```python
from build123d import *

# Parameters (mm, degrees)
BASE_FLANGE1_DEPTH    = 1
EDGE_FLANGE2_DEPTH    = 85
EDGE_FLANGE3_DEPTH    = 192.5
EDGE_FLANGE1_DEPTH    = 65
EDGE_FLANGE4_DEPTH    = 77.781745931
EDGE_FLANGE5_DEPTH    = 30
BREAK_CORNER1_START   = 128
BREAK_CORNER1_DEPTH   = 69
BREAK_CORNER1_START_2 = 196
BREAK_CORNER1_2_DEPTH = 1
BREAK_CORNER1_START_3 = -150.492424049
BREAK_CORNER1_3_DEPTH = 1
BREAK_CORNER1_START_4 = -2
BREAK_CORNER1_4_DEPTH = 19
BREAK_CORNER1_START_5 = 16
BREAK_CORNER1_5_DEPTH = 1
BREAK_CORNER1_6_DEPTH = 1
BREAK_CORNER1_START_6 = -1
BREAK_CORNER1_7_DEPTH = 1
CUT_EXTRUDE1_REACH    = 150.327


# Read off the part's stored shape, not the designer's step: Break-Corner1
# Sheet-metal steps are written as plain solids
with BuildPart() as part:
    # Sketch1 → Base-Flange1 (new body)
    with BuildSketch(Plane.XY):
        Polygon((0, 130), (-70, 130), (-70, 140), (-15, 195), (15, 195), (15, 130), (15, 0), (0, 0), align=None)
    extrude(amount=-BASE_FLANGE1_DEPTH)

    # Edge-Flange2 section (across the edge) → Edge-Flange2 (add)
    with BuildSketch(Plane(origin=(-1, 2.5, -1), x_dir=(1, 0, 0), z_dir=(0, 1, 0))):
        with BuildLine():
            Line((-1, 1), (-1, 12))
            Line((-1, 12), (0, 12))
            Line((0, 12), (0, 1))
            ThreePointArc((0, 1), (0.292893219, 0.292893219), (1, 0))
            Line((1, 0), (1, -1))
            ThreePointArc((1, -1), (-0.414213562, -0.414213562), (-1, 1))
        make_face()
    extrude(amount=EDGE_FLANGE2_DEPTH)

    # Edge-Flange3 section (across the edge) → Edge-Flange3 (add)
    with BuildSketch(Plane(origin=(16, 195, -1), x_dir=(-1, 0, 0), z_dir=(0, -1, 0))):
        with BuildLine():
            Line((-1, 1), (-1, 10))
            Line((-1, 10), (0, 10))
            Line((0, 10), (0, 1))
            ThreePointArc((0, 1), (0.292893219, 0.292893219), (1, 0))
            Line((1, 0), (1, -1))
            ThreePointArc((1, -1), (-0.414213562, -0.414213562), (-1, 1))
        make_face()
    extrude(amount=EDGE_FLANGE3_DEPTH)

    # Edge-Flange1 section (across the edge) → Edge-Flange1 (add)
    with BuildSketch(Plane(origin=(-2.5, 129, -1), x_dir=(0, 1, 0), z_dir=(-1, 0, 0))):
        with BuildLine():
            Line((-1, 1), (-1, 15.122069622))
            Line((-1, 15.122069622), (0, 15.122069622))
            Line((0, 15.122069622), (0, 1))
            ThreePointArc((0, 1), (0.292893219, 0.292893219), (1, 0))
            Line((1, 0), (1, -1))
            ThreePointArc((1, -1), (-0.414213562, -0.414213562), (-1, 1))
        make_face()
    extrude(amount=EDGE_FLANGE1_DEPTH)

    # Edge-Flange4 section (across the edge) → Edge-Flange4 (add)
    with BuildSketch(Plane(origin=(-70.707106781, 140.707106781, -1), x_dir=(0.7071067811865439, -0.7071067811865512, -3.4914813388431337e-15), z_dir=(0.7071067811865512, 0.7071067811865439, 0))):
        with BuildLine():
            Line((-1, 1), (-1, 10))
            Line((-1, 10), (0, 10))
            Line((0, 10), (0, 1))
            ThreePointArc((0, 1), (0.292893219, 0.292893219), (1, 0))
            Line((1, 0), (1, -1))
            ThreePointArc((1, -1), (-0.414213562, -0.414213562), (-1, 1))
        make_face()
    extrude(amount=EDGE_FLANGE4_DEPTH)

    # Edge-Flange5 section (across the edge) → Edge-Flange5 (add)
    with BuildSketch(Plane(origin=(-15, 196, -1), x_dir=(0, -1, 0), z_dir=(1, 0, 0))):
        with BuildLine():
            Line((-1, 1), (-1, 10))
            Line((-1, 10), (0, 10))
            Line((0, 10), (0, 1))
            ThreePointArc((0, 1), (0.292893219, 0.292893219), (1, 0))
            Line((1, 0), (1, -1))
            ThreePointArc((1, -1), (-0.414213562, -0.414213562), (-1, 1))
        make_face()
    extrude(amount=EDGE_FLANGE5_DEPTH)

    # Break-Corner1 outline → Break-Corner1 (cut)
    with BuildSketch(Plane(origin=(0, 0, 0), x_dir=(1, 0, 0), z_dir=(0, 1, 0)).offset(BREAK_CORNER1_START)):
        with BuildLine():
            ThreePointArc((-67.5, 13.622069622), (-66.767766953, 15.389836575), (-65, 16.122069622))
            Line((-65, 16.122069622), (-67.5, 16.122069622))
            Line((-67.5, 16.122069622), (-67.5, 13.622069622))
        make_face()
        with BuildLine():
            ThreePointArc((-5, 16.122069622), (-3.232233047, 15.389836575), (-2.5, 13.622069622))
            Line((-2.5, 13.622069622), (-2.5, 16.122069622))
            Line((-2.5, 16.122069622), (-5, 16.122069622))
        make_face()
        with BuildLine():
            Line((15, 11), (12.5, 11))
            ThreePointArc((12.5, 11), (14.267766953, 10.267766953), (15, 8.5))
            Line((15, 8.5), (15, 11))
        make_face()
    extrude(amount=BREAK_CORNER1_DEPTH, mode=Mode.SUBTRACT)

    # Break-Corner1 2 outline → Break-Corner1 2 (cut)
    with BuildSketch(Plane(origin=(0, 0, 0), x_dir=(1, 0, 0), z_dir=(0, 1, 0)).offset(BREAK_CORNER1_START_2)):
        with BuildLine():
            Line((-15, 11), (-15, 8.5))
            ThreePointArc((-15, 8.5), (-14.267766953, 10.267766953), (-12.5, 11))
            Line((-12.5, 11), (-15, 11))
        make_face()
    extrude(amount=BREAK_CORNER1_2_DEPTH, mode=Mode.SUBTRACT)

    # Break-Corner1 3 outline → Break-Corner1 3 (cut)
    with BuildSketch(Plane(origin=(0, 0, 0), x_dir=(0.7071067811865509, 0.707106781186544, 0), z_dir=(0.707106781186544, -0.707106781186551, 0)).offset(BREAK_CORNER1_START_3)):
        with BuildLine():
            Line((49.497474683, -11), (51.997474683, -11))
            ThreePointArc((51.997474683, -11), (50.22970773, -10.267766953), (49.497474683, -8.5))
            Line((49.497474683, -8.5), (49.497474683, -11))
        make_face()
        with BuildLine():
            ThreePointArc((127.279220614, -8.5), (126.546987567, -10.267766953), (124.779220614, -11))
            Line((124.779220614, -11), (127.279220614, -11))
            Line((127.279220614, -11), (127.279220614, -8.5))
        make_face()
    extrude(amount=BREAK_CORNER1_3_DEPTH, mode=Mode.SUBTRACT)

    # Break-Corner1 4 outline → Break-Corner1 4 (cut)
    with BuildSketch(Plane.YZ.offset(BREAK_CORNER1_START_4)):
        with BuildLine():
            ThreePointArc((195, -8.5), (194.267766953, -10.267766953), (192.5, -11))
            Line((192.5, -11), (195, -11))
            Line((195, -11), (195, -8.5))
        make_face()
        with BuildLine():
            ThreePointArc((87.449489743, -11), (86.58113883, -12.436491673), (85, -13))
            Line((85, -13), (87.5, -13))
            Line((87.5, -13), (87.5, -11))
            Line((87.5, -11), (87.449489743, -11))
        make_face()
        with BuildLine():
            Line((2.5, -13), (5, -13))
            ThreePointArc((5, -13), (3.232233047, -12.267766953), (2.5, -10.5))
            Line((2.5, -10.5), (2.5, -13))
        make_face()
    extrude(amount=BREAK_CORNER1_4_DEPTH, mode=Mode.SUBTRACT)

    # Break-Corner1 5 outline → Break-Corner1 5 (cut)
    with BuildSketch(Plane.YZ.offset(BREAK_CORNER1_START_5)):
        with BuildLine():
            Line((2.550510257, -11), (5, -11))
            ThreePointArc((5, -11), (3.232233047, -10.267766953), (2.5, -8.5))
            Line((2.5, -8.5), (2.5, -10.5))
            ThreePointArc((2.5, -10.5), (2.512659617, -10.751272405), (2.550510257, -11))
        make_face()
    extrude(amount=BREAK_CORNER1_5_DEPTH, mode=Mode.SUBTRACT)

    # Break-Corner1 6 outline → Break-Corner1 6 (cut)
    with BuildSketch(Plane.YZ.offset(BREAK_CORNER1_START_4)):
        with BuildLine():
            ThreePointArc((87.5, -10.5), (87.487340383, -10.751272405), (87.449489743, -11))
            Line((87.449489743, -11), (87.5, -11))
            Line((87.5, -11), (87.5, -10.5))
        make_face()
    extrude(amount=BREAK_CORNER1_6_DEPTH, mode=Mode.SUBTRACT)

    # Break-Corner1 7 outline → Break-Corner1 7 (cut)
    with BuildSketch(Plane.XY.offset(BREAK_CORNER1_START_6)):
        with BuildLine():
            ThreePointArc((-67.5, 130), (-69.267766953, 130.732233047), (-70, 132.5))
            Line((-70, 132.5), (-70, 130))
            Line((-70, 130), (-67.5, 130))
        make_face()
        with BuildLine():
            Line((0, 0), (2.5, 0))
            ThreePointArc((2.5, 0), (0.732233047, 0.732233047), (0, 2.5))
            Line((0, 2.5), (0, 0))
        make_face()
        with BuildLine():
            ThreePointArc((15, 2.5), (14.267766953, 0.732233047), (12.5, 0))
            Line((12.5, 0), (15, 0))
            Line((15, 0), (15, 2.5))
        make_face()
    extrude(amount=BREAK_CORNER1_7_DEPTH, mode=Mode.SUBTRACT)

    # Sketch15 → Cut-Extrude1 (cut, up to next)
    with BuildSketch(Plane(origin=(0, 129, 0), x_dir=(1, 0, 0), z_dir=(0, 1, 0)), mode=Mode.PRIVATE) as cut_extrude1_sk1:
        with BuildLine():
            Line((-60, 10.872069622), (-10, 10.872069622))
            ThreePointArc((-10, 10.872069622), (-8.25, 9.122069622), (-10, 7.372069622))
            Line((-10, 7.372069622), (-60, 7.372069622))
            ThreePointArc((-60, 7.372069622), (-61.75, 9.122069622), (-60, 10.872069622))
        make_face()
    cut_extrude1_tool1 = extrude(cut_extrude1_sk1.sketch, amount=-CUT_EXTRUDE1_REACH, mode=Mode.PRIVATE) & part.part
    add(cut_extrude1_tool1.solids().sort_by_distance((-35, 129, -9.12207))[0], mode=Mode.SUBTRACT)


solid = part.part
```
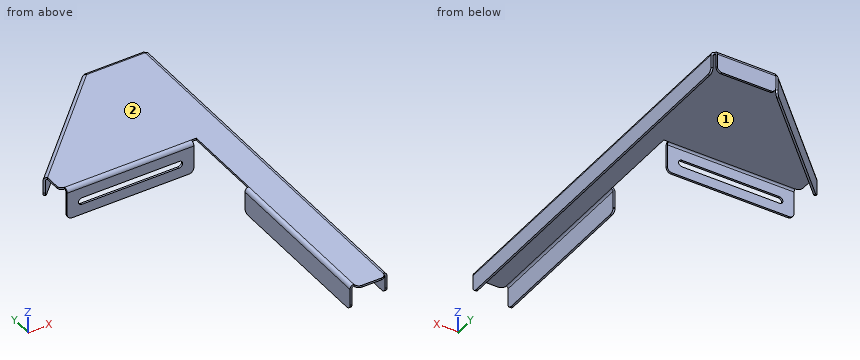
Model file for the job. Use its own axes, mm. Face numbers are marked on the shaded views. Coordinates: 2 decimals unless noted, no trailing zeros. Order: outer loops, then holes, each group sorted by start corner. A loop starts at its lowest first (then second) coordinate and runs counter-clockwise, first axis right, second up. Notation, with made-up numbers: (34, 30.25) -> (38, 30.25) arc R13 cw to (38, 53.25) -> close; hole circle Ø3 at (43.25, 1). An arc over 180 degrees is marked (long way). Return JSON: item names as keys, results as strings.
Item 1: Wall check: line 1 along X through (y, z) = (31, -5.5); line 2 along Y through (x, z) = (-52.5, -15.5); line 3 along Y through (x, z) = (-65.5, -1.5). Give the ranges that are in metal, low to high. Write a range as from..to.
Model answer:
{"line 1": "x = -2..-1, 16..17", "line 2": "y = 128..129", "line 3": "y = 128.06..129.13, 145.72..147.24"}
Item 2: Pin check, flat tips, straight feed: P1, Ø0.6, axis at y = 196, z = -4.5, coming from the -X side; P2, Ø4, axis at x = -30.5, z = -9, coming from the +Y side; P3, Ø7, axis at x = -38, z = -8, coming from the -Y side. Stop position of each tip, or through.
Model answer:
{"P1": "stops at x = -17.13", "P2": "stops at y = 184.33", "P3": "stops at y = 128"}
Item 3: Mould opens along X. For the marked faces 1 and 2 say: pulls with the +X half, pulls with the -X half, needs draft (parallel to the pull), parting line crosses it, or undercut.
Model answer:
{"face 1": "undercut", "face 2": "needs draft"}
Item 4: Slice it at A-A (x = 10). Write the cut outline in (y, z).
Model answer:
{"outline": "(0, -1) -> (195, -1) arc R1 cw to (196, -2) -> (196, -11) -> (197, -11) -> (197, -2) arc R2 ccw to (195, 0) -> (0, 0) -> close"}
Item 5: Slice it at B-B (y = 93). Write the cut outline in (x, z).
Model answer:
{"outline": "(0, -1) -> (15, -1) arc R1 cw to (16, -2) -> (16, -11) -> (17, -11) -> (17, -2) arc R2 ccw to (15, 0) -> (0, 0) -> close"}
